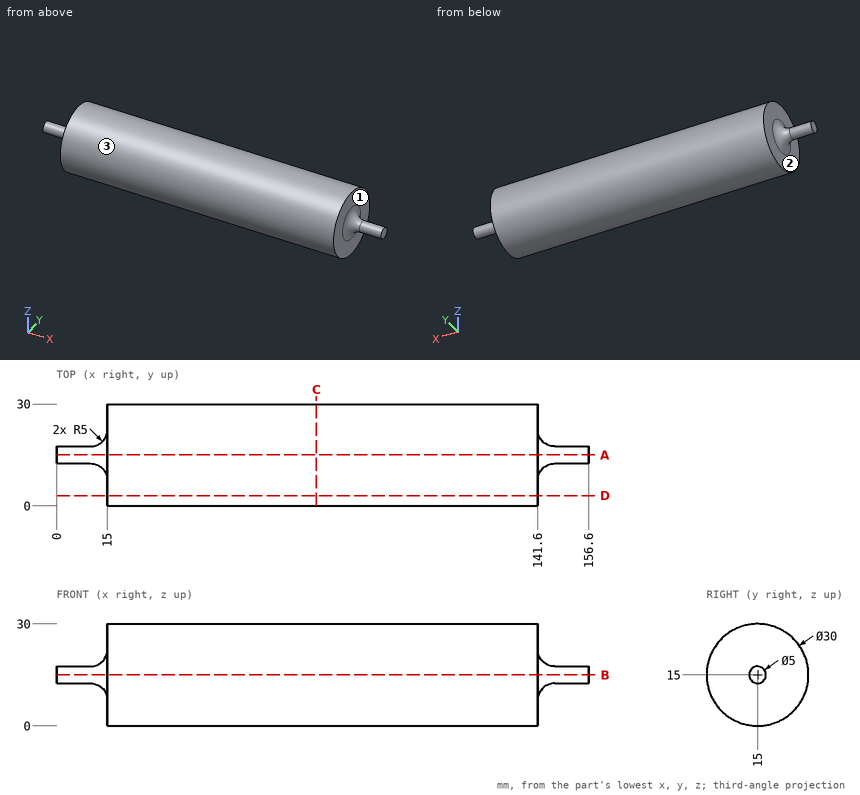
Geometry: see drawing. Coordinates: mm, zero at the bounding-box minimum. A direction names the side the tool comes from. Give positions to 0.01 mm unless a question says otherwise; leave off trailing zeros. Loops run counter-clockwise (first coordinate to the right, second up) from the corner with the lowest first, then second, coordinate; pieces in that order, holes last. Notation, with made-up numbers: (-1.5, 81.25) -> (34.5, 81.25) arc R22 ccw to (34.5, 117.25) -> close; hole circle Ø10 at (11.5, 23). An arc over 180 degrees is marked (long way). Answer as a JSON object with one key per item and string values. Group by question number.
Item 1: Pin query (flat end, axial travel): P1, Ø6, axis at y = 7.5, z = 16.5, coming from the +X side; P2, Ø4, axis at x = 51.5, y = 3.5, coming from the +Z side; P3, Ø12, axis at y = 18.5, z = 5, coming from the -X side. Return the tip coordinate at first contact, or that it passes through.
Item 2: Line query: probe 1 along X at (y, z) = (4.75, 20); probe 2 along Y at (x, z) = (28.5, 28); probe 3 along Z at (x, y) = (63.5, 15). Output: solid intervals per line, ascending.
Item 3: Cut plane A-A, the plane y = 15. Return the cut outline in (x, z), and give its area (3 significant figures).
Item 4: Cut plane D-D, the plane y = 3. Return the cut outline in (x, z), and give its area (3 significant figures).
Item 5: Reachability of the marked faces 1, 2 and 3 from +Z, -Z, +X, -X, +Y, -Y: full face, straight path, thin tool, end or side. Return the list, or none.
Item 6: Cut plane C-C, the plane x = 76.5. Return the cut outline in (y, z), and give its area (3 significant figures).
Checks:
{
 "1": {"P1": "stops at x = 142.49", "P2": "stops at z = 26.61", "P3": "stops at x = 14.07"},
 "2": {"probe 1": "x = 15 to 141.6", "probe 2": "y = 7.52 to 22.48", "probe 3": "z = 0 to 30"},
 "3": {"outline": "(0, 12.5) -> (10, 12.5) arc R5 cw to (15, 7.5) -> (15, 0) -> (141.6, 0) -> (141.6, 7.5) arc R5 cw to (146.6, 12.5) -> (156.6, 12.5) -> (156.6, 17.5) -> (146.6, 17.5) arc R5 cw to (141.6, 22.5) -> (141.6, 30) -> (15, 30) -> (15, 22.5) arc R5 cw to (10, 17.5) -> (0, 17.5) -> close", "area": "3,970 mm²"},
 "4": {"outline": "(15, 6) -> (141.6, 6) -> (141.6, 24) -> (15, 24) -> close", "area": "2,280 mm²"},
 "5": {"face 1": "+X", "face 2": "-X", "face 3": "+X, -X"},
 "6": {"outline": "circle Ø30 at (15, 15)", "area": "707 mm²"}
}
